The listing builds one solid part. Answer for the finished solid, in the listing's coordinates (mm). Face numbers are marked on the shaded views. A direction names the side the tool comes from. Round coordinates to 2 decimals unless told otherwise and drop trailing zeros. Order: outer loops, then holes, each group sorted by start corner. A loop starts at its lowest first (then second) coordinate and runs counter-clockwise, first axis right, second up. Notation, with made-up numbers: (58.5, 1.5) - (113.5, 1.5) arc R18 cw to (113.5, 36.5) - close; hole circle Ø2 at (0, 20.25). An arc over 180 degrees is marked (long way). Write item = value, one per line.
from build123d import *

# Parameters (mm, degrees)
F1_DEPTH  = 10
F2_R      = 1.5
F3_DEPTH  = 25
F6_DEPTH  = 10
F7_R      = 1.5
F8_DEPTH  = 25
F10_DEPTH = 6


with BuildPart() as f1:
    # F0 (on Front) → F1 (new body)
    with BuildSketch(Plane.XZ):
        Polygon((0, 50), (0, 0), (6, 0), (6, 19), (11, 15), (11, 0), (14, 0), (14, 19), (6, 25.4), (6, 50), align=None)
    extrude(amount=F1_DEPTH)

    # F2 (on face) → F3 (cut)
    with BuildSketch(Plane.YZ.offset(14)):
        with Locations((-5, 16)):
            Circle(F2_R)
    extrude(amount=-F3_DEPTH, mode=Mode.SUBTRACT)

    # F5 (on offset) → F6 (join)
    with BuildSketch(Plane.XY.offset(30)):
        Polygon((0, 0), (6, 0), (6, 8.978372), (14, 20.178372), (14, 30), (11, 30), (11, 22), (6, 15), (6, 30), (0, 30), align=None)
    extrude(amount=F6_DEPTH)

    # F7 (on face) → F8 (cut)
    with BuildSketch(Plane.YZ.offset(14)):
        with Locations((23.178372, 35)):
            Circle(F7_R)
    extrude(amount=-F8_DEPTH, mode=Mode.SUBTRACT)

    # F9 (on Right) → F10 (join)
    with BuildSketch(Plane.YZ):
        with BuildLine():
            Line((-7.065495, 76.976999), (-7.383263, 78.951594))
            ThreePointArc((-7.383263, 78.951594), (-5.224579, 49.143817), (-2.174402, 78.873598))
            Line((-2.174402, 78.873598), (-2.551148, 76.909403))
            ThreePointArc((-2.551148, 76.909403), (-5.194635, 51.143593), (-7.065495, 76.976999))
        make_face()
    extrude(amount=F10_DEPTH)


solid = f1.part
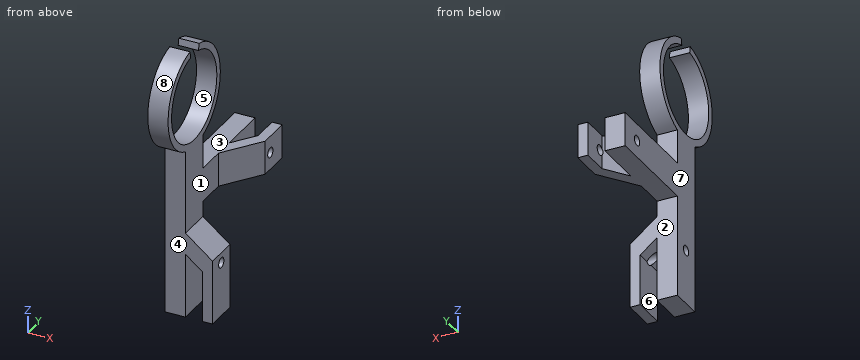
Q1. Determine the mould class of the marked faces 6, 7 and 8 for opening direction X: released by +X, released by -X, zero draft, split by the parting line, or undercut.
Model answer:
face_6 = undercut
face_7 = released by -X
face_8 = zero draft
Q2. Section D-D on z = 35 is taken. Determine the outline of the cut face in (x, y), then the cut area to 3 significant figures.
Model answer:
outline = (0, -10) - (6, -10) - (6, 8.98) - (14, 20.18) - (14, 21.68) - (10.77, 21.68) - (6, 15) - (6, 21.68) - (0, 21.68) - close; (0, 24.68) - (6, 24.68) - (6, 30) - (0, 30) - close; (11, 24.68) - (14, 24.68) - (14, 30) - (11, 30) - close
area = 279 mm^2
Q3. Flat-ended cylindrical pins translate along their axes: P1, Ø1.5, axis at x = 8.5, y = -10.5, coming from the -Z side; P2, Ø5, axis at x = 2, z = 44.5, coming from the +Y side; P3, Ø8, axis at y = 10, z = 66.5, coming from the +X side. Find the tip coordinate at first contact, or state that the pin passes through.
Model answer:
P1 = 16.55
P2 = 0
P3 = 6
Q4. Section B-B on z = 7.5 is taken. Determine the outline of the cut face in (x, y).
Model answer:
outline = (0, -10) - (6, -10) - (6, 0) - (0, 0) - close; (11, -10) - (14, -10) - (14, 0) - (11, 0) - close
Q5. Section C-C on y = -5 is taken. Determine the outline of the cut face in (x, z) (3 decimals).
Model answer:
outline = (0, 0) - (6, 0) - (6, 14.5) - (0, 14.5) - close; (0, 17.5) - (6, 17.5) - (6, 19) - (7.875, 17.5) - (14, 17.5) - (14, 19) - (6, 25.4) - (6, 51.142) - (0, 51.142) - close; (11, 0) - (14, 0) - (14, 14.5) - (11, 14.5) - close
Q6. For the marked faces 1, 2, 3, 4 and 5, determine the directions among +Z, -Z, +X, -X, +Y, -Y from which every point of the face is accessible in a straight line to the end or side of a thin tool.
Model answer:
face_1 = +Z, +X, -Y
face_2 = -Z, +X, -X, +Y
face_3 = +X, -X, +Y
face_4 = -Z, +X, -X, -Y
face_5 = +X, -X
Q7. Section A-A on x = 12.5 is taken. Determine the outline of the cut face in (y, z).
Model answer:
outline = (-10, 0) - (0, 0) - (0, 20.2) - (-10, 20.2) - close; (18.08, 30) - (30, 30) - (30, 40) - (18.08, 40) - close; hole circle Ø3 at (-5, 16); hole circle Ø3 at (23.18, 35)
Q8. Find the intervals of material crossed by line 1 (Z direction, x = 4.2, y = -5); line 2 (Z direction, x = 1, y = 2); line 3 (Z direction, x = 5, y = 15.5), in increasing order. Write a range as from..to.
Model answer:
line_1 = 0..14.5, 17.5..51.14
line_2 = 30..40, 50.88..53.19, 75.1..77.41
line_3 = 30..40
